The listing builds one solid part. Answer for the finished solid, in the listing's coordinates (mm). Face numbers are marked on the shaded views. A direction names the side the tool comes from. Coordinates: 2 decimals unless noted, no trailing zeros. Order: outer loops, then holes, each group sorted by start corner. A loop starts at its lowest first (then second) coordinate and runs counter-clockwise, first axis right, second up. Notation, with made-up numbers: M 53.25,-25.5 L 77.25,-25.5 A13 ccw 77.25,-19.5 Z; hole C 53,33.5 d1. An arc over 180 degrees is marked long. One line per item, written item: value. Start each with the question number.
Q1. Straight lines are drawn through the part: line 1 along Z through (x, y) = (2.5, 88); line 2 along X through (y, z) = (25, -10); line 3 along X through (y, z) = (170.15, -14.2). For each, find the intervals that lie inside material, in ascending order. Write a range as [from, to].
Q2. Determine the mould class of the marked faces 1, 2, 3 and 4 for opening direction X: pulls with the +X half, pulls with the -X half, needs draft (parallel to the pull), parting line crosses it, or undercut.
Q3. The part is cut by section B-B on y = 180.5. Give the vertices of the cut face in (x, z).
Q4. This flat-tipped pin is pushed along its axis until it touches: pin 1 Ø2.5 at (x, y) = (7.5, 150.15) entering from +Z. Where does it stop, or does it pass through?
Q5. For the marked faces 5 and 6, determine the directions among +Z, -Z, +X, -X, +Y, -Y from which every point of the face is accessible in a straight line to the end or side of a thin tool.
Q6. The part is cut by section A-A on z = -6.5. Give the vertices of the cut face in (x, y).
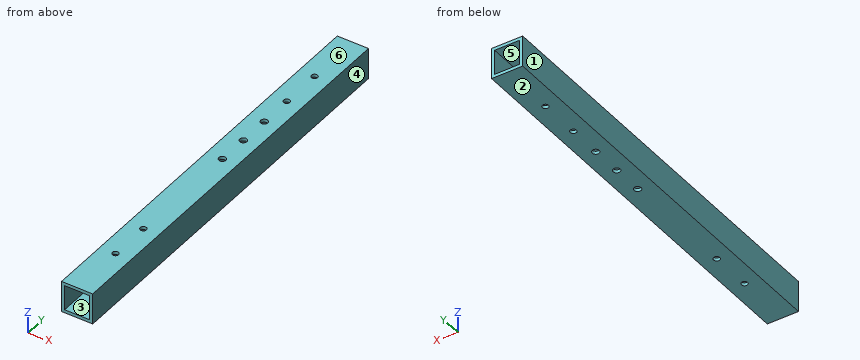
```python
from build123d import *

# Parameters (mm, degrees)
SKETCH_1_W          = 15
SKETCH_1_H          = 15
SKETCH_1_W_2        = 12
SKETCH_1_H_2        = 12
EXTRUDE_1_DEPTH     = 197.65
SKETCH_2_R          = 1.5
SKETCH_2_R_2        = 1.7
CUT_EXTRUDE_1_DEPTH = 199.785116395


with BuildPart() as part:
    # 草图1 → 凸台-拉伸1 (new body)
    with BuildSketch(Plane(origin=(0, 0, 0), x_dir=(1, 0, 0), z_dir=(0, 1, 0))):
        with Locations((7.5, 7.5)):
            Rectangle(SKETCH_1_W, SKETCH_1_H)
        with Locations((7.5, 7.5)):
            Rectangle(SKETCH_1_W_2, SKETCH_1_H_2, mode=Mode.SUBTRACT)
    extrude(amount=EXTRUDE_1_DEPTH)

    # 草图2 (on Front Plane) → 切除-拉伸1 (cut, through all)
    with BuildSketch(Plane.XY):
        with Locations((7.5, 47.5)):
            Circle(SKETCH_2_R)
        with Locations((7.5, 27.5)):
            Circle(SKETCH_2_R)
        with Locations((7.7, 103.825)):
            Circle(SKETCH_2_R_2)
        with Locations((7.7, 118.825)):
            Circle(SKETCH_2_R_2)
        with Locations((7.7, 133.825)):
            Circle(SKETCH_2_R_2)
        with Locations((7.5, 150.15)):
            Circle(SKETCH_2_R)
        with Locations((7.5, 170.15)):
            Circle(SKETCH_2_R)
    extrude(amount=-CUT_EXTRUDE_1_DEPTH, mode=Mode.SUBTRACT)


solid = part.part
```
Output:
1. line 1: z = [-15, -13.5], [-1.5, 0]
1. line 2: x = [0, 1.5], [13.5, 15]
1. line 3: x = [0, 6], [9, 15]
2. face 1: pulls with the -X half
2. face 2: needs draft
2. face 3: undercut
2. face 4: pulls with the +X half
3. outline: M 0,-15 L 15,-15 L 15,0 L 0,0 Z; hole M 1.5,-13.5 L 13.5,-13.5 L 13.5,-1.5 L 1.5,-1.5 Z
4. pin 1: passes through
5. face 5: +Y, -Y
5. face 6: +Z, +X, -X, +Y, -Y
6. outline: M 0,0 L 1.5,0 L 1.5,197.65 L 0,197.65 Z; M 13.5,0 L 15,0 L 15,197.65 L 13.5,197.65 Z
